Part print with two shaded views. Sizes in mm from the minimum x, y, z corner. Round coordinates to 2 decimals unless told otherwise and drop trailing zeros. Loops run counter-clockwise (first coordinate to the right, second up) from the corner with the lowest first, then second, coordinate; pieces in that order, holes last. Notation, with made-up numbers: (-8.75, 73.5) - (3.25, 73.5) arc R18 cw to (3.25, 104.5) - close; hole circle Ø11 at (-12.5, 3). An arc over 180 degrees is marked (long way). Use a Markdown table: item, result.
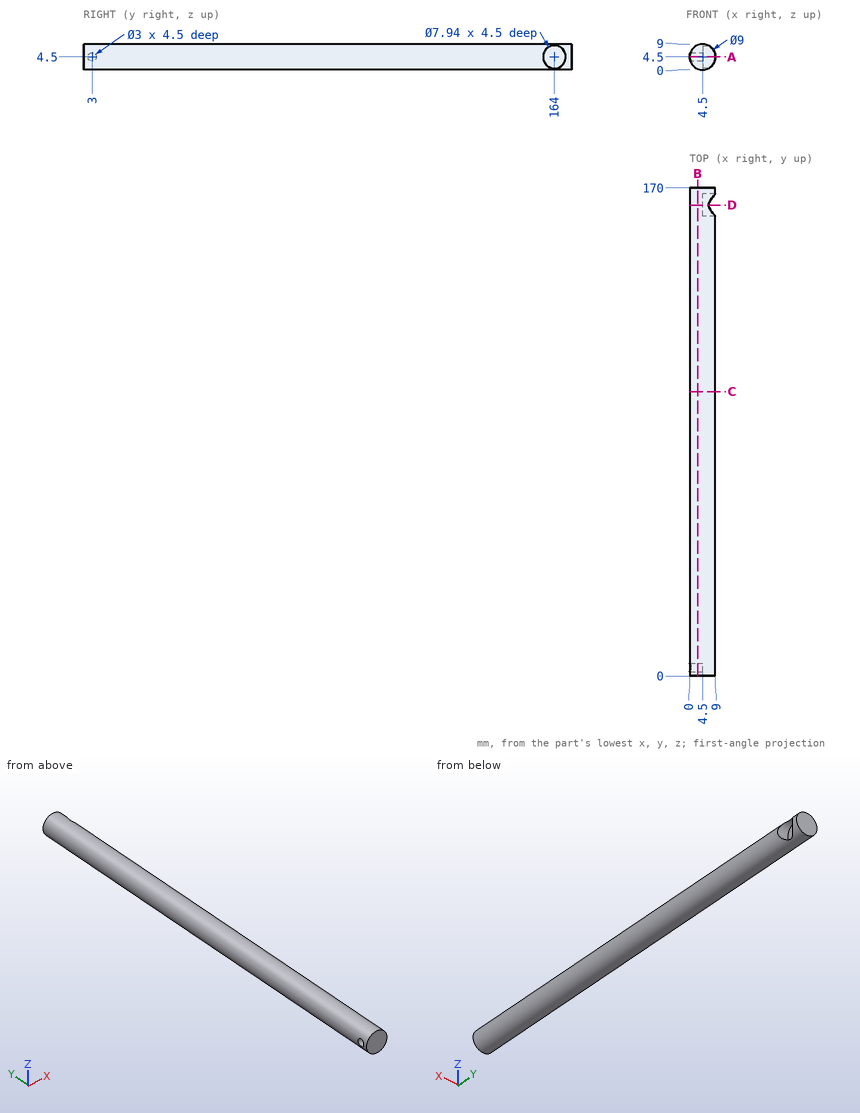
Q1. Cut at C-C, the plane y = 99. List the corners of the cut face in (x, z).
Results found:
| item | result |
|---|---|
| outline | circle Ø9 at (4.5, 4.5) |
Q2. Cut at A-A, the plane z = 4.5. List the corners of the cut face in (x, y), plus the area to 3 significant figures.
Results found:
| item | result |
|---|---|
| outline | (0, 0) - (9, 0) - (9, 160.03) - (4.5, 160.03) - (4.5, 167.97) - (9, 167.97) - (9, 170) - (0, 170) - (0, 4.5) - (4.5, 4.5) - (4.5, 1.5) - (0, 1.5) - close |
| area | 1,480 mm2 |
Q3. Cut at B-B, the plane x = 2.75. List the corners of the cut face in (y, z), plus the area to 3 significant figures.
Results found:
| item | result |
|---|---|
| outline | (0, 0.35) - (170, 0.35) - (170, 8.65) - (0, 8.65) - close; hole circle Ø3 at (3, 4.5) |
| area | 1,400 mm2 |
Q4. Probe line 1 (Y direction, x = 2.95, z = 4.5); line 2 (Y direction, x = 6.5, z = 4); line 3 (X direction, y = 153, z = 5). List the from-to ranges inside material, lowest first.
Results found:
| item | result |
|---|---|
| line 1 | y = 0 to 1.5, 4.5 to 170 |
| line 2 | y = 0 to 160.06, 167.94 to 170 |
| line 3 | x = 0.03 to 8.97 |
Q5. Cut at D-D, the plane y = 164. List the corners of the cut face in (x, z), plus the area to 3 significant figures.
Results found:
| item | result |
|---|---|
| outline | (4.5, 0.53) - (4.5, 8.47) - (6.62, 8.47) arc R4.5 ccw (long way) to (6.62, 0.53) - close |
| area | 33.3 mm2 |
Q6. Drop flat-ended pins along their axis: pin 1 (2.5 mm diameter, centred on y = 164, z = 3, fed in from +X); pin 2 (1 mm diameter, centred on y = 131, z = 2, fed in from -X); pin 3 (1.5 mm diameter, centred on y = 3.5, z = 5, fed in from -X). Give the stop position or say it passes through.
Results found:
| item | result |
|---|---|
| pin 1 | stops at x = 4.5 |
| pin 2 | stops at x = 0.47 |
| pin 3 | stops at x = 4.5 |
